from build123d import *
from OCP.BRepFilletAPI import BRepFilletAPI_MakeFillet

# Parameters (mm, degrees)
CROQUIS1_W              = 40
CROQUIS1_H              = 60
SALIENTE_EXTRUIR1_DEPTH = 13
CROQUIS19_W             = 5.497004625
CROQUIS19_H             = 49.49
CORTAR_EXTRUIR6_DEPTH   = 40
CROQUIS17_R             = 1.5
CORTAR_EXTRUIR8_DEPTH   = 40
CROQUIS20_W             = 5
CROQUIS20_H             = 44
CORTAR_EXTRUIR11_DEPTH  = 40
CROQUIS23_W             = 28
CROQUIS23_H             = 10.7
CORTAR_EXTRUIR12_DEPTH  = 60.5
CROQUIS24_R             = 2.75
CORTAR_EXTRUIR13_DEPTH  = 40
REDONDEO2_R1            = 2.5
REDONDEO2_R2            = 5
CROQUIS25_W             = 2
CROQUIS25_H             = 13
CORTAR_EXTRUIR15_DEPTH  = 10.51
MATRIZC1_COUNT          = 2
CROQUIS27_W             = 2
CROQUIS27_H             = 7.52
CORTAR_EXTRUIR16_DEPTH  = 5.5
CROQUIS28_W             = 2
CROQUIS28_H             = 7.52
CORTAR_EXTRUIR17_DEPTH  = 5.5
CROQUIS29_W             = 2
CROQUIS29_H             = 9.681242813
CORTAR_EXTRUIR18_DEPTH  = 3


with BuildPart() as part:
    # Croquis1 → Saliente-Extruir1 (new body)
    with BuildSketch(Plane.XY):
        Rectangle(CROQUIS1_W, CROQUIS1_H)
    extrude(amount=SALIENTE_EXTRUIR1_DEPTH)

    # Croquis19 → Cortar-Extruir6 (cut)
    with BuildSketch(Plane(origin=(20, 0, 0), x_dir=(0, 0, -1), z_dir=(1, 0, 0))):
        with Locations((-10.251497688, -5.255)):
            Rectangle(CROQUIS19_W, CROQUIS19_H)
    extrude(amount=-CORTAR_EXTRUIR6_DEPTH, mode=Mode.SUBTRACT)

    # Croquis17 → Cortar-Extruir8 (cut)
    with BuildSketch(Plane(origin=(20, 0, 0), x_dir=(0, 0, -1), z_dir=(1, 0, 0))):
        with Locations((-5, -27.27)):
            Circle(CROQUIS17_R)
    extrude(amount=-CORTAR_EXTRUIR8_DEPTH, mode=Mode.SUBTRACT)

    # Croquis20 → Cortar-Extruir11 (cut)
    with BuildSketch(Plane(origin=(20, 0, 0), x_dir=(0, 0, -1), z_dir=(1, 0, 0))):
        with Locations((-5.002995375, -2.5)):
            Rectangle(CROQUIS20_W, CROQUIS20_H)
    extrude(amount=-CORTAR_EXTRUIR11_DEPTH, mode=Mode.SUBTRACT)

    # Croquis23 → Cortar-Extruir12 (cut)
    with BuildSketch(Plane(origin=(0, 30, 0), x_dir=(1, 0, 0), z_dir=(0, 1, 0))):
        with Locations((0, -7.85)):
            Rectangle(CROQUIS23_W, CROQUIS23_H)
    extrude(amount=-CORTAR_EXTRUIR12_DEPTH, mode=Mode.SUBTRACT)

    # Croquis24 → Cortar-Extruir13 (cut)
    with BuildSketch(Plane(origin=(20, 0, 0), x_dir=(0, 0, -1), z_dir=(1, 0, 0))):
        with Locations((-8, 24.5)):
            Circle(CROQUIS24_R)
    extrude(amount=-CORTAR_EXTRUIR13_DEPTH, mode=Mode.SUBTRACT)

    # Redondeo2: one fillet with a radius per group of edges: ONE call of the kernel's fillet builder (fillet() takes one radius for all edges)
    redondeo2_edges_1 = [part.edges().sort_by_distance(p)[0] for p in [
        (17, -24.5, 7.502995375),
        (17, -30, 7.502995375),
        (-17, -30, 7.502995375),
        (-17, -24.5, 7.502995375),
    ]]
    redondeo2_edges_2 = [part.edges().sort_by_distance(p)[0] for p in [
        (17, 19.49, 13),
        (17, 30, 13),
        (-17, 19.49, 13),
        (-17, 30, 13),
    ]]
    redondeo2 = BRepFilletAPI_MakeFillet(part.part.solid().wrapped)
    for e in redondeo2_edges_1:
        redondeo2.Add(REDONDEO2_R1, e.wrapped)
    for e in redondeo2_edges_2:
        redondeo2.Add(REDONDEO2_R2, e.wrapped)
    add(Compound.cast(redondeo2.Shape()), mode=Mode.REPLACE)

    # Croquis25 → Cortar-Extruir15 (cut)
    with BuildSketch(Plane(origin=(0, 30, 0), x_dir=(1, 0, 0), z_dir=(0, 1, 0))):
        with Locations((19, -6.5)):
            Rectangle(CROQUIS25_W, CROQUIS25_H)
    cortar_extruir15 = extrude(amount=-CORTAR_EXTRUIR15_DEPTH, mode=Mode.SUBTRACT)

    # MatrizC1: Cortar-Extruir15 ×2 about axis
    matrizc1_axis = Axis((0, 26.946865888, 5), (0, -1, 0))
    for i in range(1, MATRIZC1_COUNT):
        add(cortar_extruir15.rotate(matrizc1_axis, i * 360 / MATRIZC1_COUNT), mode=Mode.SUBTRACT)

    # Croquis27 → Cortar-Extruir16 (cut)
    with BuildSketch(Plane.XZ.offset(30)):
        with Locations((19, 3.76)):
            Rectangle(CROQUIS27_W, CROQUIS27_H)
    extrude(amount=-CORTAR_EXTRUIR16_DEPTH, mode=Mode.SUBTRACT)

    # Croquis28 → Cortar-Extruir17 (cut)
    with BuildSketch(Plane.XZ.offset(30)):
        with Locations((-19, 3.76)):
            Rectangle(CROQUIS28_W, CROQUIS28_H)
    extrude(amount=-CORTAR_EXTRUIR17_DEPTH, mode=Mode.SUBTRACT)

    # Croquis29 → Cortar-Extruir18 (cut)
    with BuildSketch(Plane(origin=(0, 0, 10), x_dir=(-1, 0, 0), z_dir=(0, 0, -1))):
        with Locations((19, 24.748045712)):
            Rectangle(CROQUIS29_W, CROQUIS29_H)
    extrude(amount=-CORTAR_EXTRUIR18_DEPTH, mode=Mode.SUBTRACT)


solid = part.part
CAD build for the part. Positions are in the model's coordinates, mm. A direction names the side the tool comes from. Give positions to 0.01 mm unless a question says otherwise; leave off trailing zeros. Loops run counter-clockwise (first coordinate to the right, second up) from the corner with the lowest first, then second, coordinate; pieces in that order, holes last. Notation, with made-up numbers: M 44.25,-35.75 L 60.25,-35.75 A21 ccw 60.25,-17.75 Z; hole C -39.5,12.25 d11. An arc over 180 degrees is marked long. Answer in a Markdown table with one row per item. Add a question column.
Item 1: Band-saw the part on D-D on z = 12.25. Give the cut face in (x, y).
Item 2: Mould opens along Y. For faces 5 (the face through (16, 19.5, 5)), 6 (the face through (17, -3, 2.503)), 7 (the face through (18, -27, 3)), 8 (the face through (0, -30, 2)) say: +Y half, -Y half, draft (parallel to the pull), parting line (faces both ways), or undercut.
Item 3: Probe probe 1 along Y at (x, z) = (-14.85, 5); probe 2 along Y at (x, z) = (16.75, 8); probe 3 along X at (y, z) = (27.5, 5). List the from-to ranges inside material, lowest first.
Item 4: Tool access for faces 1 (the face through (15.97, -25.25, 6.79)), 2 (the face through (19, 19.49, 1)), 3 (the face through (-14, 20, 7)), 4 (the face through (-18, -27, 3)): list every direction of +Z, -Z, +X, -X, +Y, -Y with a clear straight run to the whole face (end or side of a thin tool).
Item 5: Drop flat-ended pins along their axis: P1, Ø5, axis at x = 16, y = 3, coming from the +Z side; P2, Ø8, axis at x = 6.5, y = 7.5, coming from the -Z side; P3, Ø3, axis at y = 23.5, z = 1.5, coming from the +X side; P4, Ø5.5, axis at y = 25, z = 5, coming from the -X side. Give the stop position or say it passes through.
Item 6: Band-saw the part on A-A on z = 1.5. Give the cut face in (x, y).
Item 7: Band-saw the part on B-B on x = 16. Give the number of separate pieces and of enclosed holes in the cut face, then the cut area to 3 significant figures.
Reply:
| question | item | result |
|---|---|---|
| 1 | outline | M -18,21.86 L -14,21.86 L -14,27.63 L -18,27.63 Z; M 14,21.86 L 18,21.86 L 18,27.63 L 14,27.63 Z |
| 2 | face 5 | undercut |
| 2 | face 6 | undercut |
| 2 | face 7 | draft |
| 2 | face 8 | -Y half |
| 3 | probe 1 | y = -30 to -28.77, -25.77 to -24.5, 19.5 to 30 |
| 3 | probe 2 | y = 19.49 to 21.75, 27.25 to 30 |
| 3 | probe 3 | x = -18 to -14, 14 to 18 |
| 4 | face 1 | +Z, +X, -X |
| 4 | face 2 | +Z, -Z, +X, +Y |
| 4 | face 3 | +Z, +Y, -Y |
| 4 | face 4 | +Z, -Z, -X, -Y |
| 5 | P1 | stops at z = 2.5 |
| 5 | P2 | stops at z = 0 |
| 5 | P3 | stops at x = 18 |
| 5 | P4 | stops at x = -18 |
| 6 | outline | M -20,-24.5 L -18,-24.5 L -18,-30 L 18,-30 L 18,-24.5 L 20,-24.5 L 20,19.49 L 18,19.49 L 18,30 L -18,30 L -18,19.49 L -20,19.49 Z |
| 7 | separate pieces | 1 |
| 7 | enclosed holes | 2 |
| 7 | area | 244 mm^2 |
